The listing builds one solid part. Answer for the finished solid, in the listing's coordinates (mm). Face numbers are marked on the shaded views. A direction names the side the tool comes from. Give positions to 0.01 mm unless a question says otherwise; leave off trailing zeros. Loops run counter-clockwise (first coordinate to the right, second up) from the corner with the lowest first, then second, coordinate; pieces in that order, holes last.
Item 1: Section B-B, the plane z = 5.75 is taken. Give the vertices of the cut face in (x, y), and give its area (3 significant figures).
Item 2: The mould has two halves that part along Z. Classify the marked faces 1, 2 and 3: pulls with the +Z half, pulls with the -Z half, needs draft (parallel to the pull), parting line crosses it, or undercut.
Item 3: Consider line 1 along X through (y, z) = (0.5, 2.5); line 2 along X through (y, z) = (0, 3.5); line 3 along Z through (x, y) = (-1.15, -1.75). Determine where each line is inside the solid, lowest interval first.
Item 4: Each of these flat-tipped pins is pushed along its axis until it touches: pin 1 Ø1.5 at (x, z) = (-0.5, 3.5) entering from -Y; pin 2 Ø1.3 at (x, y) = (-2, -1) entering from +Z. Where does it stop, or does it pass through?
Item 5: Section D-D, the plane y = -0.25 is taken. Give the vertices of the cut face in (x, z), and give its area (3 significant figures).
Item 6: A tool of negligible diameter and unlimited length cuts with its end or side. For the marked faces 4, 5 and 6, from which of +Z, -Z, +X, -X, +Y, -Y can it reach the whole face along a straight path? Write none if from no direction.
Item 7: Section C-C, the plane y = -3 is taken. Give the vertices of the cut face in (x, z).
Item 8: Section A-A, the plane x = -2.5 is taken. Give the vertices of the cut face in (y, z).
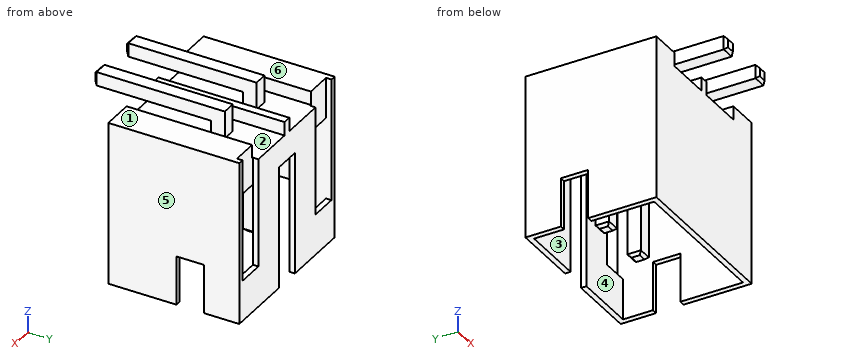
from build123d import *

# Parameters (mm, degrees)
SKETCH_1_W           = 6
SKETCH_1_H           = 4.8
SKETCH_1_W_2         = 5.6
SKETCH_1_H_2         = 4.4
EXTRUDE_1_DEPTH      = 6
SKETCH_2_W           = 5.6
SKETCH_2_H           = 4.4
EXTRUDE_1_2_DEPTH    = 1.5
SKETCH_3_W           = 1
SKETCH_3_H           = 4.5
CUT_EXTRUDE_1_DEPTH  = 0.2
SKETCH_4_W           = 1.8
SKETCH_4_H           = 1
CUT_EXTRUDE_2_DEPTH  = 9.818163074
SKETCH_5_W           = 0.5
SKETCH_5_H           = 0.5
EXTRUDE_2_DEPTH      = 3.7
SKETCH_7_W           = 1.7
SKETCH_7_H           = 4.8
CUT_EXTRUDE_3_DEPTH  = 0.5
EXTRUDE_3_DEPTH      = 0.5
EXTRUDE_3_DEPTH_BACK = 0.5
SKETCH_6_W           = 0.5
SKETCH_6_H           = 0.5
SKETCH_8_W           = 0.5
SKETCH_8_H           = 0.5
EXTRUDE_4_DEPTH      = 4.8
CHAMFER_1_SIZE       = 0.1


with BuildPart() as part:
    # 草图1 → Extrude 1 (new body)
    with BuildSketch(Plane.XY):
        Rectangle(SKETCH_1_W, SKETCH_1_H)
        Rectangle(SKETCH_1_W_2, SKETCH_1_H_2, mode=Mode.SUBTRACT)
    extrude(amount=EXTRUDE_1_DEPTH)

    # 草图2 → Extrude 1 2 (add)
    with BuildSketch(Plane.XY.offset(6)):
        Rectangle(SKETCH_2_W, SKETCH_2_H)
    extrude(amount=-EXTRUDE_1_2_DEPTH)

    # 草图3 → 切除-拉伸1 (cut)
    with BuildSketch(Plane(origin=(0, 2.4, 0), x_dir=(1, 0, 0), z_dir=(0, 1, 0))):
        Polygon((0, 0), (0.5, 0), (0.5, -4.5), (-0.5, -4.5), (-0.5, 0), align=None)
        with Locations((-2.3, -3.75)):
            Rectangle(SKETCH_3_W, SKETCH_3_H)
        with Locations((2.3, -3.75)):
            Rectangle(SKETCH_3_W, SKETCH_3_H)
    extrude(amount=-CUT_EXTRUDE_1_DEPTH, mode=Mode.SUBTRACT)

    # 草图4 → 切除-拉伸2 (cut, through all)
    with BuildSketch(Plane.ZY.offset(3)):
        with Locations((0.9, 0.6)):
            Rectangle(SKETCH_4_W, SKETCH_4_H)
    extrude(amount=-CUT_EXTRUDE_2_DEPTH, mode=Mode.SUBTRACT)

    # 草图5 → 凸台-拉伸2 (add)
    with BuildSketch(Plane(origin=(0, 0, 4.5), x_dir=(-1, 0, 0), z_dir=(0, 0, -1))):
        with Locations((-1, 0.6)):
            Rectangle(SKETCH_5_W, SKETCH_5_H)
        with Locations((1, 0.6)):
            Rectangle(SKETCH_5_W, SKETCH_5_H)
    extrude(amount=EXTRUDE_2_DEPTH)

    # 草图7 → 切除-拉伸3 (cut)
    with BuildSketch(Plane.XY.offset(6)):
        with Locations((-1, 0)):
            Rectangle(SKETCH_7_W, SKETCH_7_H)
        with Locations((1, 0)):
            Rectangle(SKETCH_7_W, SKETCH_7_H)
    extrude(amount=-CUT_EXTRUDE_3_DEPTH, mode=Mode.SUBTRACT)

    # 草图6 → 凸台-拉伸3 (add, two sides: drawn at the far end of the back side and taken through both)
    with BuildSketch(Plane.XY.offset(6).offset(-EXTRUDE_3_DEPTH_BACK)):
        with Locations((-1, 0.6)):
            Rectangle(SKETCH_6_W, SKETCH_6_H)
        with Locations((1, 0.6)):
            Rectangle(SKETCH_6_W, SKETCH_6_H)
    extrude(amount=EXTRUDE_3_DEPTH + EXTRUDE_3_DEPTH_BACK)

    # 草图8 → 凸台-拉伸4 (add)
    with BuildSketch(Plane(origin=(0, 0.85, 0), x_dir=(1, 0, 0), z_dir=(0, 1, 0))):
        with Locations((-1, -6.25)):
            Rectangle(SKETCH_8_W, SKETCH_8_H)
        with Locations((1, -6.25)):
            Rectangle(SKETCH_8_W, SKETCH_8_H)
    extrude(amount=-EXTRUDE_4_DEPTH)

    # 倒角1
    chamfer_1_edges = [part.edges().sort_by_distance(p)[0] for p in [
        (0.75, 0.6, 0.8),
        (1, 0.85, 0.8),
        (1.25, 0.6, 0.8),
        (1, 0.35, 0.8),
        (-1.25, 0.6, 0.8),
        (-1, 0.85, 0.8),
        (-0.75, 0.6, 0.8),
        (-1, 0.35, 0.8),
        (-1.25, -3.95, 6.25),
        (-1, -3.95, 6),
        (-0.75, -3.95, 6.25),
        (-1, -3.95, 6.5),
        (0.75, -3.95, 6.25),
        (1, -3.95, 6),
        (1.25, -3.95, 6.25),
        (1, -3.95, 6.5),
    ]]
    chamfer(chamfer_1_edges, length=CHAMFER_1_SIZE)


solid = part.part
Worked answers:
1. outline: (-3, -2.4) - (-1.85, -2.4) - (-1.85, 2.2) - (-2.8, 2.2) - (-2.8, 2.4) - (-3, 2.4) - close; (-1.25, 0.35) - (-0.75, 0.35) - (-0.75, 0.85) - (-1.25, 0.85) - close; (-0.15, -2.4) - (0.15, -2.4) - (0.15, 2.4) - (-0.15, 2.4) - close; (0.75, 0.35) - (1.25, 0.35) - (1.25, 0.85) - (0.75, 0.85) - close; (1.85, -2.4) - (3, -2.4) - (3, 2.4) - (2.8, 2.4) - (2.8, 2.2) - (1.85, 2.2) - close
1. area: 12.6 mm2
2. face 1: pulls with the +Z half
2. face 2: undercut
2. face 3: needs draft
3. line 1: x = -3 to -2.8, -1.25 to -0.75, 0.75 to 1.25, 2.8 to 3
3. line 2: x = -3 to -2.8, 2.8 to 3
3. line 3: z = 4.5 to 5.5, 6 to 6.5
4. pin 1: stops at y = -2.4
4. pin 2: stops at z = 6
5. outline: (-3, 0) - (-2.8, 0) - (-2.8, 4.5) - (2.8, 4.5) - (2.8, 0) - (3, 0) - (3, 6) - (1.85, 6) - (1.85, 5.5) - (0.15, 5.5) - (0.15, 6) - (-0.15, 6) - (-0.15, 5.5) - (-1.85, 5.5) - (-1.85, 6) - (-3, 6) - close; (-1.25, 6) - (-0.75, 6) - (-0.75, 6.5) - (-1.25, 6.5) - close; (0.75, 6) - (1.25, 6) - (1.25, 6.5) - (0.75, 6.5) - close
5. area: 9.60 mm2
6. face 4: -Z
6. face 5: +Z, -Z, +X, +Y, -Y
6. face 6: +Z, -X, +Y, -Y
7. outline: (-1.25, 6) - (-0.75, 6) - (-0.75, 6.5) - (-1.25, 6.5) - close; (0.75, 6) - (1.25, 6) - (1.25, 6.5) - (0.75, 6.5) - close
8. outline: (-2.4, 0) - (-2.2, 0) - (-2.2, 4.5) - (2.2, 4.5) - (2.2, 6) - (-2.4, 6) - close; (2.2, 0) - (2.4, 0) - (2.4, 1.5) - (2.2, 1.5) - close
